```python
from build123d import *

# Parameters (mm, degrees)
SKETCH1_W                      = 106
SKETCH1_H                      = 84
BOSS_EXTRUDE1_DEPTH            = 30
SKETCH2_W                      = 11
SKETCH2_H                      = 25
CUT_EXTRUDE1_DEPTH             = 104.754517974
M3_CLEARANCE_HOLE1_D           = 3.4
M3_CLEARANCE_HOLE1_DEPTH       = 10
M3_CLEARANCE_HOLE1_CSINK_D     = 3.45
M3_CLEARANCE_HOLE1_CSINK_ANGLE = 90
M3_CLEARANCE_HOLE1_TIP         = 1.021463052
M3_CLEARANCE_HOLE2_D           = 3.4
M3_CLEARANCE_HOLE2_CSINK_D     = 3.45
M3_CLEARANCE_HOLE2_CSINK_ANGLE = 90


with BuildPart() as part:
    # Sketch1 → Boss-Extrude1 (new body)
    with BuildSketch(Plane(origin=(0, 0, 0), x_dir=(1, 0, 0), z_dir=(0, 1, 0))):
        Rectangle(SKETCH1_W, SKETCH1_H)
    extrude(amount=BOSS_EXTRUDE1_DEPTH)

    # Sketch2 → Cut-Extrude1 (cut, through all)
    with BuildSketch(Plane.XY.offset(42)):
        with Locations((47.5, 17.5)):
            Rectangle(SKETCH2_W, SKETCH2_H)
        with Locations((-47.5, 17.5)):
            Rectangle(SKETCH2_W, SKETCH2_H)
    extrude(amount=-CUT_EXTRUDE1_DEPTH, mode=Mode.SUBTRACT)

    # M3 Clearance Hole1
    with Locations(Plane(origin=(0, 30, 0), x_dir=(1, 0, 0), z_dir=(0, 1, 0))):
        with Locations((-34, 34), (34, 34), (34, -34), (-34, -34)):
            CounterSinkHole(M3_CLEARANCE_HOLE1_D / 2, M3_CLEARANCE_HOLE1_CSINK_D / 2, depth=M3_CLEARANCE_HOLE1_DEPTH, counter_sink_angle=M3_CLEARANCE_HOLE1_CSINK_ANGLE)
            with Locations((0, 0, -(M3_CLEARANCE_HOLE1_DEPTH + M3_CLEARANCE_HOLE1_TIP / 2))):  # 118° drill point
                Cone(0, M3_CLEARANCE_HOLE1_D / 2, M3_CLEARANCE_HOLE1_TIP, mode=Mode.SUBTRACT)

    # M3 Clearance Hole2 (through all)
    with Locations(Plane(origin=(0, 5, 0), x_dir=(1, 0, 0), z_dir=(0, 1, 0))):
        with Locations((-47.5, 0), (47.5, 0)):
            CounterSinkHole(M3_CLEARANCE_HOLE2_D / 2, M3_CLEARANCE_HOLE2_CSINK_D / 2, counter_sink_angle=M3_CLEARANCE_HOLE2_CSINK_ANGLE)


solid = part.part
```
Design review of the part built by this model. Coordinates are the model's own, in mm. A direction names the side the tool comes from. Give positions to 0.01 mm unless a question says otherwise; leave off trailing zeros. Order: outer loops, then holes, each group sorted by start corner. A loop starts at its lowest first (then second) coordinate and runs counter-clockwise, first axis right, second up. Notation, with made-up numbers: (31.25, 87) -> (36.25, 87) arc R33 cw to (36.25, 120) -> close; hole circle Ø4 at (84, 84). An arc over 180 degrees is marked (long way). Write each question's results on one line, items separated by ' | '. Start each with the question number.
Q1. Add section C-C on y = 7.25. Give the boundary of the cut face in (x, z), and give its area (3 significant figures).
Q2. Mouldability with a two-part tool opening along X and no side actions: class faces 1 (the flat face through (42, 17, 1)), 2 (the conical face through (-34.038, 19.156, -34.293)), 3 (the flat face through (-1, 30, -1)) as +X half, -X half, draft (parallel to the pull), parting line (faces both ways), or undercut.
Q3. Machinability: for faces 4 (the flat face through (50, 5, 1)), 5 (the conical face through (33.962, 19.156, -34.293)), 6 (the flat face through (-45, 5, 1)), which of the approach directions +Z, -Z, +X, -X, +Y, -Y give a long, thin tool a straight path to every point of the face, cutting with its end or side? Answer none if there is none.
Q4. For pin 1 (7.5 mm diameter, centred on y = 18.5, z = -1.5, fed in from +X); pin 2 (4.5 mm diameter, centred on x = -47.5, z = 0, fed in from +Y); pin 3 (3 mm diameter, centred on x = 34, z = 34, fed in from +Y), all flat-tipped, find the tip position at first contact; note any pin that passes through.
Q5. Wall thickness on L1, parallel to X at y = 25.5, z = 34; L2, parallel to Z at x = 47.5, y = 2.8: over which ranges is each line inside the solid? List them lowest first. Write a range as from..to.
Q6. Add section A-A on x = 47.5. Give the boundary of the cut face in (y, z) (3 decimals), and give its area (3 significant figures).
Q7. Add section B-B on z = 0. Give the boundary of the cut face in (x, y) (3 decimals).
Found:
1) outline: (-42, -42) -> (42, -42) -> (42, 42) -> (-42, 42) -> close | area: 7,060 mm2
2) face 1: +X half | face 2: undercut | face 3: draft
3) face 4: +Z, -Z, +X, +Y | face 5: +Y | face 6: +Z, -Z, -X, +Y
4) pin 1: stops at x = 42 | pin 2: stops at y = 5 | pin 3: stops at y = 19.88
5) L1: x = -42..-35.7, -32.3..32.3, 35.7..42 | L2: z = -42..-1.7, 1.7..42
6) outline: (0, -42) -> (5, -42) -> (5, -1.725) -> (4.975, -1.7) -> (0, -1.7) -> close; (0, 1.7) -> (4.975, 1.7) -> (5, 1.725) -> (5, 42) -> (0, 42) -> close | area: 403 mm2
7) outline: (-53, 0) -> (-49.2, 0) -> (-49.2, 4.975) -> (-49.225, 5) -> (-53, 5) -> close; (-45.8, 0) -> (45.8, 0) -> (45.8, 4.975) -> (45.775, 5) -> (42, 5) -> (42, 30) -> (-42, 30) -> (-42, 5) -> (-45.775, 5) -> (-45.8, 4.975) -> close; (49.2, 0) -> (53, 0) -> (53, 5) -> (49.225, 5) -> (49.2, 4.975) -> close
